Here's how the part is built. I have some questions about the finished solid (model axes, mm). A direction names the side the tool comes from. Give positions to 0.01 mm unless a question says otherwise; leave off trailing zeros. Write each loop counter-clockwise with the first axis right and the second up, starting at its lowest first coordinate (ties: lowest second). Pieces come first, ordered by that corner, then holes. Notation, with made-up numbers: (88, 76.5) - (109, 76.5) arc R25 cw to (109, 99.5) - close; hole circle Ø5 at (37, 42). An arc over 180 degrees is marked (long way). Write each question's results on one line, items separated by ' | '. Start each with the question number.
Item 1: Which directions (+Z, -Z, +X, -X, +Y, -Y) give clear straight access to the entire face, cutting with the end or side of a thin tool? Please do faces 1 (the flat face through (42, -28.006, 13)), 2 (the flat face through (-25, -28.006, 13)), 3 (the flat face through (13, 41.562, -23)).
Item 2: Suppose I cut it at B-B on x = -5. List the corners of the cut face in (y, z) for me.
Item 3: Suppose I cut it at C-C on z = -6. List the corners of the cut face in (x, y) for me.
Item 4: Suppose I cut it at A-A on y = 34. List the corners of the cut face in (x, z) for me.
Item 5: Please list where these lines run through material, in increasing order: line 1 along X through (y, z) = (9.5, -37); line 2 along Y through (x, z) = (48, 15.5).
Item 6: Will these pins go through, and if not, where does the flat tip stop? P1, Ø8, axis at y = 6.5, z = -21.5, coming from the -X side; P2, Ø7.5, axis at x = 12.5, z = -17, coming from the +Y side; P3, Ø7.5, axis at x = -14.5, z = 10, coming from the -Y side; P4, Ø2, axis at x = 26.5, z = -19, coming from the -Y side.
```python
from build123d import *

# Parameters (mm, degrees)
F0_W     = 109.44755
F0_H     = 70.106957
F1_DEPTH = 25.4
F2_W     = 69.736343
F2_H     = 70.670309
F3_DEPTH = 25.4
F4_W     = 109.896999
F4_H     = 70.047663
F5_DEPTH = 2.032


with BuildPart() as f1:
    # F0 (on Top) → F1 (new body)
    with BuildSketch(Plane.XY):
        with Locations((4.438201, 7.047662)):
            Rectangle(F0_W, F0_H)
    extrude(amount=F1_DEPTH)

    # F2 (on Right) → F3 (join)
    with BuildSketch(Plane.YZ):
        with Locations((6.693443, -9.806676)):
            Rectangle(F2_W, F2_H)
    extrude(amount=F3_DEPTH)

    # F4 (on Top) → F5 (join)
    with BuildSketch(Plane.XY):
        with Locations((4.825505, 7.471751)):
            Rectangle(F4_W, F4_H)
    extrude(amount=F5_DEPTH)


solid = f1.part
```
Checked values:
1) face 1: +Z, -Z, +X, -Y | face 2: +Z, -Z, -X, -Y | face 3: -Z, +X, -X, +Y
2) outline: (-28.01, 0) - (42.5, 0) - (42.5, 2.03) - (42.1, 2.03) - (42.1, 25.4) - (-28.01, 25.4) - close
3) outline: (0, -28.17) - (25.4, -28.17) - (25.4, 41.56) - (0, 41.56) - close
4) outline: (-50.29, 0) - (0, 0) - (0, -45.14) - (25.4, -45.14) - (25.4, 0) - (59.77, 0) - (59.77, 2.03) - (59.16, 2.03) - (59.16, 25.4) - (25.4, 25.4) - (25.4, 25.53) - (0, 25.53) - (0, 25.4) - (-50.29, 25.4) - close
5) line 1: x = 0 to 25.4 | line 2: y = -28.01 to 42.1
6) P1: stops at x = 0 | P2: stops at y = 41.56 | P3: stops at y = -28.01 | P4: passes through
